Input: dimensioned drawing with shaded views. Units: mm. Origin: part minimum x, y, z. A direction names the side the tool comes from. Give positions to 0.01 mm unless a question says otherwise; leave off trailing zeros. Write each loop counter-clockwise with the first axis right and the second up, starting at its lowest first coordinate (ties: lowest second). Pieces come first, ordered by that corner, then holes. Notation, with made-up numbers: (28.5, 12) -> (54.5, 12) arc R22 ccw to (54.5, 39) -> close; hole circle Ø7 at (66, 82.5). An arc over 180 degrees is marked (long way). Answer as a JSON object with one key per item and string values.
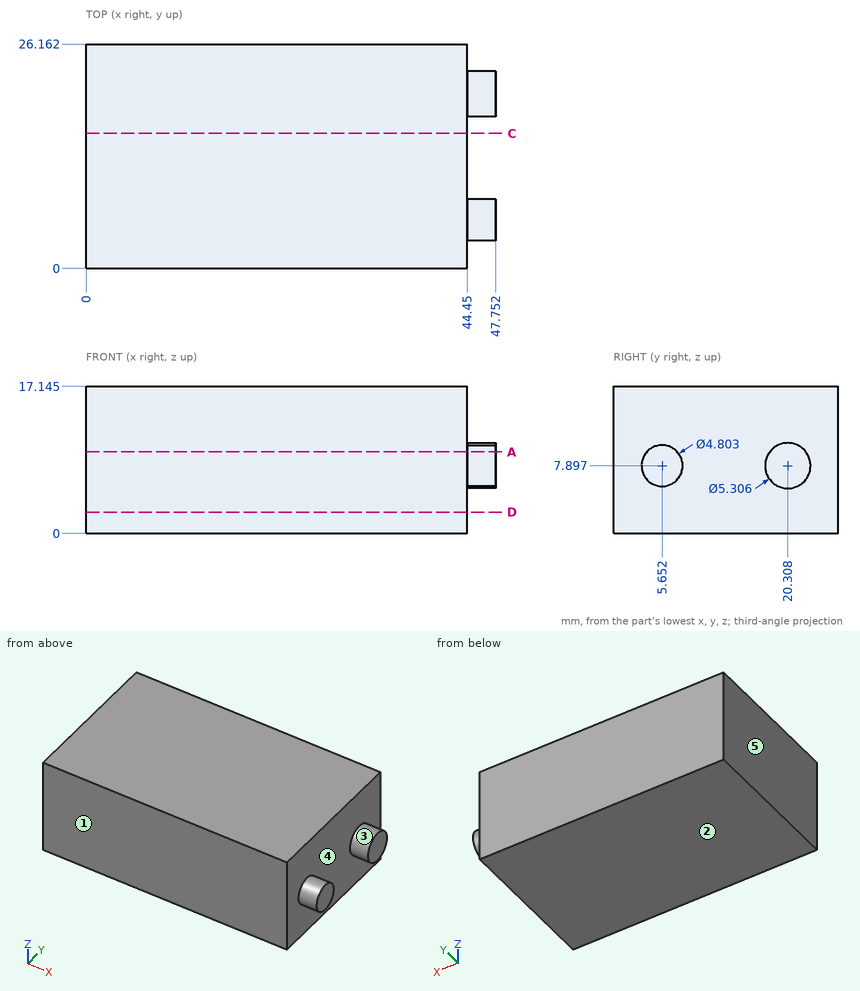
Q1. First-contact query: P1, Ø3, axis at y = 10, z = 3, coming from the +X side. Flat tip, straight axial feed; report the tip coordinate or a pass-through.
Values:
{"P1": "x = 44.45"}
Q2. Mould query, pull axis Y, two halves, no side actions, for the marked faces 1, 2 and 3. Classes: pulls with the +Y half, pulls with the -Y half, needs draft (parallel to the pull), parting line crosses it, or undercut.
Values:
{"face 1": "pulls with the -Y half", "face 2": "needs draft", "face 3": "undercut"}
Q3. Set-up query: the marked faces 4 and 5. Return all of +Z, -Z, +X, -X, +Y, -Y with unobstructed straight access to the full face (end or side cutting, diameter ignored); none if empty.
Values:
{"face 4": "+X", "face 5": "+Z, -Z, -X, +Y, -Y"}
Q4. Cut plane D-D (z = 2.5). Return the cut outline in (x, y).
Values:
{"outline": "(0, 0) -> (44.45, 0) -> (44.45, 26.16) -> (0, 26.16) -> close"}
Q5. Cut plane C-C (y = 15.75). Return the cut outline in (x, z) (3 decimals), and give its area (3 significant figures).
Values:
{"outline": "(0, 0) -> (44.45, 0) -> (44.45, 17.145) -> (0, 17.145) -> close", "area": "762 mm²"}
Q6. Cut plane A-A (z = 9.5). Return the cut outline in (x, y), and give its area (3 significant figures).
Values:
{"outline": "(0, 0) -> (44.45, 0) -> (44.45, 3.86) -> (47.75, 3.86) -> (47.75, 7.44) -> (44.45, 7.44) -> (44.45, 18.19) -> (47.75, 18.19) -> (47.75, 22.42) -> (44.45, 22.42) -> (44.45, 26.16) -> (0, 26.16) -> close", "area": "1,190 mm²"}
Q7. Material intervals for L1, parallel to X at y = 7.75, z = 5, sorted ascending. Write a range as from..to.
Values:
{"L1": "0..44.45"}
